Read the model definition and answer for the solid it produces. Units are mm, in the model's axes. Coordinates: 2 decimals unless noted, no trailing zeros. Write each loop counter-clockwise with the first axis right and the second up, starting at its lowest first coordinate (ties: lowest second). Pieces come first, ordered by that corner, then holes.
Item 1: Section A-A (z = 0.6) is taken. State how many separate pieces and enclosed holes the cut face has, then the cut area to 3 significant figures.
Item 2: Straight lines are drawn through the part: probe 1 along Y at (x, z) = (85, 1.45); probe 2 along Y at (x, z) = (36, 0.2). For each, find the intervals that lie inside material, in ascending order.
Item 3: Section B-B (x = 0) is taken. Give the vertices of the cut face in (y, z), then the cut area to 3 significant figures.
Item 4: Section C-C (x = 59.5) is taken. Give the vertices of the cut face in (y, z).
Item 5: Determine the mould class of faces 1 (the face through (13.4, -0.07, 1.48)), 2 (the face through (47, 0, 3)), 3 (the face through (47, 5, 1)) for opening direction Y: released by +Y, released by -Y, zero draft, split by the parting line, or undercut.
Autodesk Fusion 360 part; units mm, degrees
sketch "Sketch1" plane through (0, 0, 0) normal (0, 0, 1) x (1, 0, 0)
  circle A0 centre (0, 0) radius 1.6
  line L0 (-5, 5) -> (100, 5)
  line L1 (100, 5) -> (100, -5)
  line L2 (100, -5) -> (-5, -5)
  line L3 (-5, -5) -> (-5, 5)
  line L4 (-5, 0) -> (100, 0) construction
  circle A1 centre (5, 0) radius 1.6
  circle A2 centre (10, 0) radius 1.6
  circle A3 centre (15, 0) radius 1.6
  circle A4 centre (20, 0) radius 1.6
  circle A5 centre (25, 0) radius 1.6
  circle A6 centre (30, 0) radius 1.6
  circle A7 centre (35, 0) radius 1.6
  circle A8 centre (40, 0) radius 1.6
  circle A9 centre (45, 0) radius 1.6
  circle A10 centre (50, 0) radius 1.6
  circle A11 centre (55, 0) radius 1.6
  circle A12 centre (60, 0) radius 1.6
  circle A13 centre (65, 0) radius 1.6
  circle A14 centre (70, 0) radius 1.6
  circle A15 centre (75, 0) radius 1.6
  circle A16 centre (80, 0) radius 1.6
  circle A17 centre (85, 0) radius 1.6
  circle A18 centre (90, 0) radius 1.6
  circle A19 centre (95, 0) radius 1.6
  dimension "d56" = 3.2
  dimension "d57" = 5
  dimension "d58" = 10
  dimension "d59" = 105
  dimension "d62" = 5
  dimension "d63" = 0
extrude "Extrude1" add sketch "Sketch1" along normal blind 3
move_body "Move1" [suppressed]
equation "d56 = HoleDiameter"
equation "d57 = HoleSpacing"
equation "d58 = LegWidth"
equation "d59 = LegsJointLength"
equation "d62 = HoleSpacing"
equation "d64 = Thickness"
equation "HoleDiameter = 3.2 mm"
equation "Thickness = 3 mm"
equation "HoleSpacing = 5 mm"
equation "LegWidth = 10 mm"
equation "LegsJointLength = 105 mm"
Established:
1. separate pieces: 1
1. enclosed holes: 20
1. area: 889 mm2
2. probe 1: y = -5 to -1.6, 1.6 to 5
2. probe 2: y = -5 to -1.25, 1.25 to 5
3. outline: (-5, 0) - (-1.6, 0) - (-1.6, 3) - (-5, 3) - close; (1.6, 0) - (5, 0) - (5, 3) - (1.6, 3) - close
3. area: 20.4 mm2
4. outline: (-5, 0) - (-1.52, 0) - (-1.52, 3) - (-5, 3) - close; (1.52, 0) - (5, 0) - (5, 3) - (1.52, 3) - close
5. face 1: undercut
5. face 2: zero draft
5. face 3: released by +Y
